CAD build for the part. Positions are in the model's coordinates, mm. Face numbers are marked on the shaded views. Coordinates: 2 decimals unless noted, no trailing zeros. Order: outer loops, then holes, each group sorted by start corner. A loop starts at its lowest first (then second) coordinate and runs counter-clockwise, first axis right, second up. Notation, with made-up numbers: M -23.5,16.5 L 16.5,16.5 A9 cw 16.5,29.5 Z; hole C 88.25,-30.5 d8. An arc over 180 degrees is marked long. One line per item, written item: value.
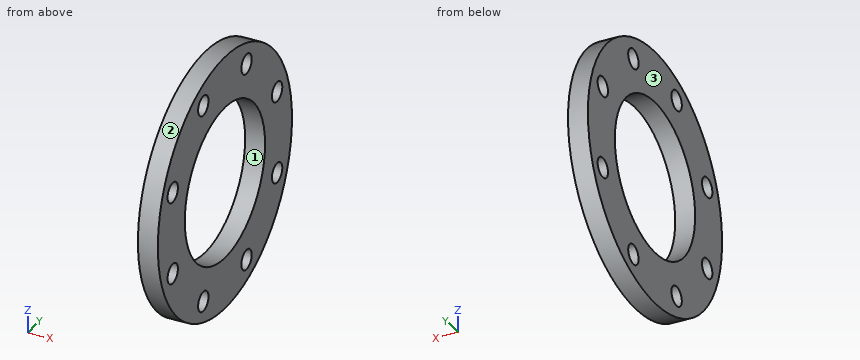
Autodesk Inventor part; units mm, degrees
ref_plane "YZ Plane" through (0, 0, 0) normal (1, 0, 0) x (0, 1, 0)
ref_plane "XZ Plane" through (0, 0, 0) normal (0, 1, 0) x (-1, 0, 0)
ref_plane "XY Plane" through (0, 0, 0) normal (0, 0, 1) x (1, 0, 0)
sketch "Sketch1" plane through (0, 0, 0) normal (0, 0, 1) x (1, 0, 0)
  line L0 (22, 142.5) -> (0, 142.5)
  line L1 (0, 142.5) -> (0, 85.25)
  line L2 (0, 85.25) -> (0, 0) construction
  line L3 (0, 0) -> (22, 0) construction
  line L4 (22, 142.5) -> (22, 85.25)
  line L5 (22, 85.25) -> (0, 85.25)
  line L6 (22, 85.25) -> (22, 0) construction
  dimension "d0" = 285
  dimension "d1" = 22
  dimension "d5" = 170.5
revolve "Revolution1" add sketch "Sketch1" angle 360 about axis through (0, 0, 0) along (1, 0, 0)
sketch "Sketch2" plane through (0, 0, 0) normal (-1, 0, 0) x (0, 0, 1)
  circle A0 centre (0, 0) radius 85.25
  line L0 (0, 120) -> (0, 0) construction
  circle A1 centre (0, 0) radius 142.5
  circle A2 centre (0, 0) radius 120 construction
  line L1 (0, 0) -> (45.922, 110.8655) construction
  circle A3 centre (45.922, 110.8655) radius 11
  dimension "d6" = 22
  dimension "d7" = 120
  dimension "d8" = 22.5
extrude "Extrusion1" cut sketch "Sketch2" against normal through all contours A3
pattern_circular "Circular Pattern1" count 8 over 360 about axis through (11, 0, 0) along (1, 0, 0) of "Extrusion1"
equation "\"d6\" = dd2"
equation "\"d7\" = 0.5 * k"
equation "\"d0\" = D"
equation "\"d1\" = b"
equation "\"d5\" = dd5"
equation "\"b\" = 22"
equation "\"D\" = 285"
equation "\"dd2\" = 22"
equation "\"dd5\" = 170.5"
equation "\"Size_Designation\" = 1.2345"
properties part number "DIN 2576 Slip-On Flange for Welding Series 1 (ISO) - PN 10 150 x 168.3" material "Steel"
Q1. Mould opens along Y. For the marked faces 1, 2 and 3 say: released by +Y, released by -Y, zero draft, split by the parting line, or undercut.
Recorded:
face 1: undercut
face 2: split by the parting line
face 3: zero draft
Q2. Slice it at C-C (y = 50). List the corners of the cut face in (x, z), plus the area to 3 significant figures.
Recorded:
outline: M 0,-133.44 L 22,-133.44 L 22,-121.08 L 0,-121.08 Z; M 0,-100.65 L 22,-100.65 L 22,-69.05 L 0,-69.05 Z; M 0,69.05 L 22,69.05 L 22,100.65 L 0,100.65 Z; M 0,121.08 L 22,121.08 L 22,133.44 L 0,133.44 Z
area: 1,930 mm^2
Q3. Slice it at A-A (z = 0). List the corners of the cut face in (x, y).
Recorded:
outline: M 0,-142.5 L 22,-142.5 L 22,-85.25 L 0,-85.25 Z; M 0,85.25 L 22,85.25 L 22,142.5 L 0,142.5 Z
Q4. Pin check, flat tips, straight feed: pin 1 Ø5 at (x, y) = (15, -20) entering from +Z; pin 2 Ø12 at (x, z) = (4.5, 76.5) entering from -Y; pin 3 Ø2 at (x, z) = (16, -101) entering from +Y. Stop position of each tip, or through.
Recorded:
pin 1: stops at z = 141.42
pin 2: stops at y = -123.84
pin 3: stops at y = 101.52
Q5. Drill centre lines: line 1 along Z through (x, y) = (3.75, -117.5); line 2 along Z through (x, y) = (11, -105); line 3 along Y through (x, z) = (5.5, 52.5). Where is each one in solid material? Low to high.
Recorded:
line 1: z = -80.62 to -54.7, -37.15 to 37.15, 54.7 to 80.62
line 2: z = -96.34 to -55.23, -36.62 to 36.62, 55.23 to 96.34
line 3: y = -132.48 to -119.68, -102.05 to -67.17, 67.17 to 102.05, 119.68 to 132.48
Q6. Slice it at D-D (x = 5). Give the number of separate pieces and of enclosed holes in the cut face, plus the area to 3 significant figures.
Recorded:
separate pieces: 1
enclosed holes: 9
area: 37,900 mm^2
